Geometry: final body of the model. Coordinates: model frame, mm. A direction names the side the tool comes from. Give positions to 0.01 mm unless a question says otherwise; leave off trailing zeros. Write each loop counter-clockwise with the first axis right and the second up, starting at its lowest first coordinate (ties: lowest second). Pieces come first, ordered by that corner, then holes. Notation, with made-up numbers: (46, 8.5) - (76, 8.5) arc R22 cw to (76, 31.5) - close; hole circle Ø7 at (-24, 14.25). An arc over 180 degrees is marked (long way). Return JSON: item names as keys, results as strings.
from build123d import *

# Parameters (mm, degrees)
EXTRUDE_1_DEPTH        = 3
FILLET_1_R             = 2
HOLE_WIZARD_M3_1_D     = 3.4
HOLE_WIZARD_M3_1_DEPTH = 7
HOLE_WIZARD_M3_1_TIP   = 1.021463052
SKETCH_10_R            = 5
EXTRUDE_2_DEPTH        = 1


with BuildPart() as part:
    # 스케치1 → 회전1 (revolve)
    with BuildSketch(Plane.XY, mode=Mode.PRIVATE) as revolve_1_sk:
        Polygon((0, 0), (13.85, 0), (13.85, 19), (10.85, 22), (3, 22), (3, 27), (1.5875, 27), (1.5875, 37), (0, 37), align=None)
    revolve(revolve_1_sk.sketch.rotate(Axis((0, 0, 0), (0, -1, 0)), 90), axis=Axis((0, 0, 0), (0, -1, 0)))

    # 스케치2 → 보스-돌출1 (add)
    with BuildSketch(Plane.XZ):
        with BuildLine():
            ThreePointArc((12.614530686, -5.718051729), (8, 0), (12.614530686, 5.718051729))
            ThreePointArc((12.614530686, 5.718051729), (9.793428919, 9.793428919), (5.718051729, 12.614530686))
            ThreePointArc((5.718051729, 12.614530686), (0, 8), (-5.718051729, 12.614530686))
            ThreePointArc((-5.718051729, 12.614530686), (-9.793428919, 9.793428919), (-12.614530686, 5.718051729))
            ThreePointArc((-12.614530686, 5.718051729), (-8, 0), (-12.614530686, -5.718051729))
            ThreePointArc((-12.614530686, -5.718051729), (-9.793428919, -9.793428919), (-5.718051729, -12.614530686))
            ThreePointArc((-5.718051729, -12.614530686), (0, -8), (5.718051729, -12.614530686))
            ThreePointArc((5.718051729, -12.614530686), (9.793428919, -9.793428919), (12.614530686, -5.718051729))
        make_face()
    extrude(amount=EXTRUDE_1_DEPTH)

    # 필렛1
    fillet_1_edges = [part.edges().sort_by_distance(p)[0] for p in [
        (-9.793428919, -3, -9.793428919),
        (9.793428919, -3, -9.793428919),
        (9.793428919, -3, 9.793428919),
        (-9.793428919, -3, 9.793428919),
    ]]
    fillet(fillet_1_edges, radius=FILLET_1_R)

    # M3 여유 구멍1
    with Locations(Plane(origin=(0, -3, 0), x_dir=(-1, 0, 0), z_dir=(0, -1, 0))):
        with Locations((5.656854249, -5.656854249), (-5.656854249, 5.656854249), (-6.717514421, -6.717514421), (6.717514421, 6.717514421)):
            Hole(HOLE_WIZARD_M3_1_D / 2, depth=HOLE_WIZARD_M3_1_DEPTH)
            with Locations((0, 0, -(HOLE_WIZARD_M3_1_DEPTH + HOLE_WIZARD_M3_1_TIP / 2))):  # 118° drill point
                Cone(0, HOLE_WIZARD_M3_1_D / 2, HOLE_WIZARD_M3_1_TIP, mode=Mode.SUBTRACT)

    # 스케치10 → 보스-돌출2 (add)
    with BuildSketch(Plane.XZ.offset(3)):
        with Locations(Location((0, 0, 0), (0, 0, 270))):
            Circle(SKETCH_10_R)
    extrude(amount=EXTRUDE_2_DEPTH)


solid = part.part
Q1. Material intervals for probe 1 along Y at (x, z) = (-2.5, 2.25); probe 2 along Y at (x, z) = (3.75, 6.75); probe 3 along X at (y, z) = (14, -11), sorted ascending. Write a range as [from, to].
Answer key:
{"probe 1": "y = [-4, 22]", "probe 2": "y = [-3, 22]", "probe 3": "x = [-8.42, 8.42]"}
Q2. Mould query, pull axis X, two halves, no side actions, for faces 6 (the cylindrical face through (7.631, 0.549, 5.284)), 7 (the cylindrical face through (-0.9, 24.54, 2.86)), 8 (the flat face through (11, 0, 0)), 9 (the conical face through (-6.854, 4.844, -6.456)). Classes: pulls with the +X half, pulls with the -X half, needs draft (parallel to the pull), parting line crosses it, or undercut.
Answer key:
{"face 6": "undercut", "face 7": "parting line crosses it", "face 8": "needs draft", "face 9": "undercut"}
Q3. Section query B-B, the plane y = 0.5. Return the cut outline in (x, z).
Answer key:
{"outline": "circle Ø27.7 at (0, 0); hole circle Ø3.4 at (-6.72, -6.72); hole circle Ø3.4 at (-5.66, 5.66); hole circle Ø3.4 at (5.66, -5.66); hole circle Ø3.4 at (6.72, 6.72)"}
Q4. Section query A-A, the plane x = 0. Return the cut outline in (y, z), plus the area to 3 significant figures.
Answer key:
{"outline": "(-4, -5) - (-3, -5) - (-3, -8) - (0, -8) - (0, -13.85) - (19, -13.85) - (22, -10.85) - (22, -3) - (27, -3) - (27, -1.59) - (37, -1.59) - (37, 1.59) - (27, 1.59) - (27, 3) - (22, 3) - (22, 10.85) - (19, 13.85) - (0, 13.85) - (0, 8) - (-3, 8) - (-3, 5) - (-4, 5) - close", "area": "720 mm^2"}
Q5. Section query D-D, the plane y = 20.5. Return the cut outline in (x, z).
Answer key:
{"outline": "circle Ø24.7 at (0, 0)"}
Q6. Set-up query: faces 1 (the cylindrical face through (3.96, 0.55, -5.73)), 2 (the cylindrical face through (-8, -1, 0)), 3 (the flat face through (0, 0, -11)), 4 (the flat face through (0, 0, 11)), 5 (the flat face through (1.3, 27, 1.3)). Return all of +Z, -Z, +X, -X, +Y, -Y with unobstructed straight access to the full face (end or side cutting, diameter ignored); none if empty.
Answer key:
{"face 1": "-Y", "face 2": "-X, -Y", "face 3": "-Z, -Y", "face 4": "+Z, -Y", "face 5": "+Y"}
Q7. Pin query (flat end, axial travel): P1, Ø5, axis at x = 9, z = -7, coming from the -Y side; P2, Ø8, axis at y = 1.5, z = 1, coming from the -X side; P3, Ø5, axis at y = 15, z = -10.5, coming from the +X side; P4, Ø12, axis at x = -10.5, y = 29.5, coming from the +Z side. Return the tip coordinate at first contact, or that it passes through.
Answer key:
{"P1": "stops at y = -3", "P2": "stops at x = -13.85", "P3": "stops at x = 11.31", "P4": "passes through"}
Q8. Section query C-C, the plane z = 0. Return the cut outline in (x, y), plus the area to 3 significant figures.
Answer key:
{"outline": "(-13.85, 0) - (-8, 0) - (-8, -3) - (-5, -3) - (-5, -4) - (5, -4) - (5, -3) - (8, -3) - (8, 0) - (13.85, 0) - (13.85, 19) - (10.85, 22) - (3, 22) - (3, 27) - (1.59, 27) - (1.59, 37) - (-1.59, 37) - (-1.59, 27) - (-3, 27) - (-3, 22) - (-10.85, 22) - (-13.85, 19) - close", "area": "720 mm^2"}
